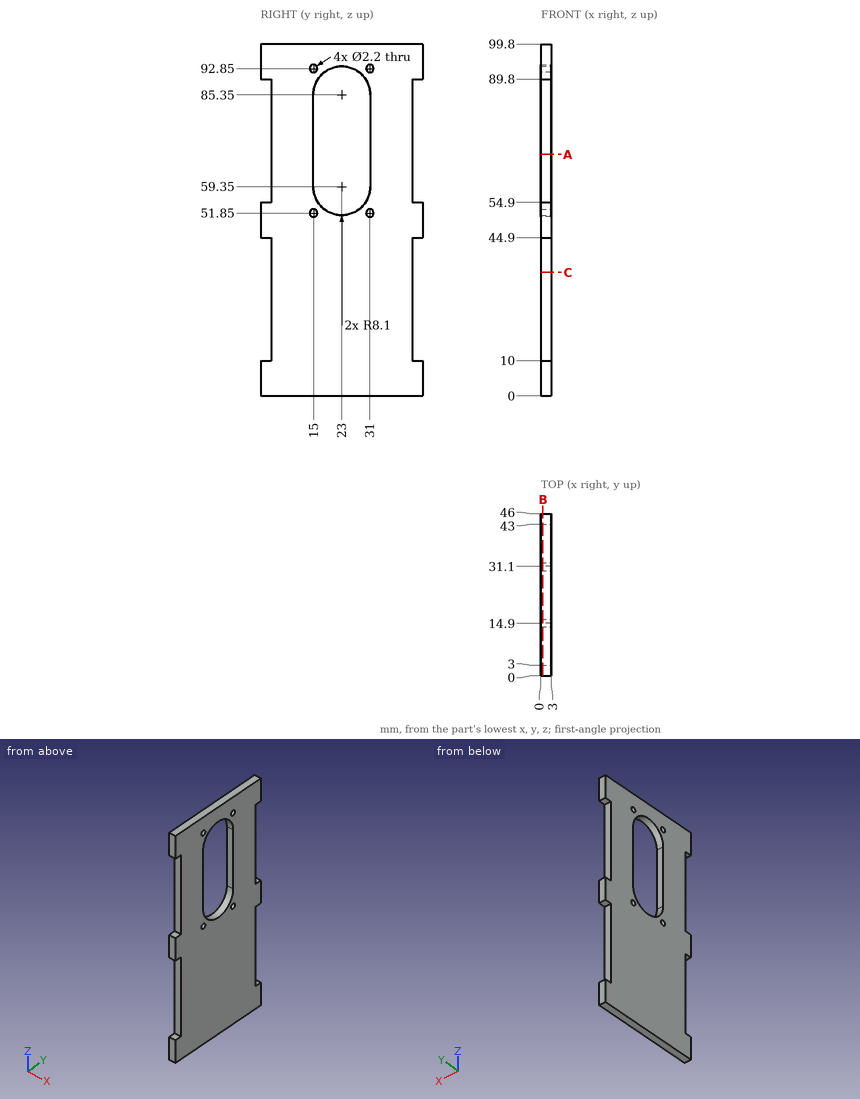
Drawing for the job (mm, zero at the part's lowest x, y, z). Round coordinates to 2 decimals unless told otherwise and drop trailing zeros. Loops run counter-clockwise (first coordinate to the right, second up) from the corner with the lowest first, then second, coordinate; pieces in that order, holes last. Notation, with made-up numbers: (63, 74.5) - (94, 74.5) arc R11 cw to (94, 80.5) - close; hole circle Ø2 at (35, 1). An arc over 180 degrees is marked (long way). Write each question's results on one line, items separated by ' | '.
(1) Saw through at A-A, the plane z = 68.5. List the corners of the cut face in (x, y), then the cut area to 3 significant figures.
Answer below:
outline: (0, 3) - (3, 3) - (3, 14.9) - (0, 14.9) - close; (0, 31.1) - (3, 31.1) - (3, 43) - (0, 43) - close | area: 71.4 mm^2
(2) Saw through at C-C, the plane z = 35. List the corners of the cut face in (x, y).
Answer below:
outline: (0, 3) - (3, 3) - (3, 43) - (0, 43) - close
(3) Saw through at B-B, the plane x = 0.6. List the corners of the cut face in (y, z).
Answer below:
outline: (0, 0) - (46, 0) - (46, 10) - (43, 10) - (43, 44.9) - (46, 44.9) - (46, 54.9) - (43, 54.9) - (43, 89.8) - (46, 89.8) - (46, 99.8) - (0, 99.8) - (0, 89.8) - (3, 89.8) - (3, 54.9) - (0, 54.9) - (0, 44.9) - (3, 44.9) - (3, 10) - (0, 10) - close; hole circle Ø2.2 at (15, 51.85); hole circle Ø2.2 at (15, 92.85); hole (14.9, 59.35) arc R8.1 ccw to (31.1, 59.35) - (31.1, 85.35) arc R8.1 ccw to (14.9, 85.35) - close; hole circle Ø2.2 at (31, 51.85); hole circle Ø2.2 at (31, 92.85)
(4) Wall check: L1, parallel to Y at x = 0.25, z = 77; L2, parallel to Y at x = 0.85, z = 92.85; L3, parallel to Y at x = 2.75, z = 30.5. Give the ranges that are in metal, low to high.
Answer below:
L1: y = 3 to 14.9, 31.1 to 43 | L2: y = 0 to 13.9, 16.1 to 19.94, 26.06 to 29.9, 32.1 to 46 | L3: y = 3 to 43
(5) Pin check, flat tips, straight feed: pin 1 (1.5 mm diameter, centred on x = 1, z = 72.5, fed in from +Y); pin 2 (1.5 mm diameter, centred on x = 1.5, z = 68, fed in from -Y). Stop position of each tip, or through.
Answer below:
pin 1: stops at y = 43 | pin 2: stops at y = 3
